```python
from build123d import *

# Parameters (mm, degrees)
CUT_EXTRUDE1_DEPTH = 1.5
CHAMFER1_SIZE      = 0.5


with BuildPart() as part:
    # Sketch2 → Revolve1 (revolve)
    with BuildSketch(Plane(origin=(0, 0, 0), x_dir=(1, 0, 0), z_dir=(0, 1, 0))):
        Polygon((-18, -4.5), (-11, -4.5), (-11, 0), (-5, 0), (-5, -5.4), (-11, -5.4), (-11, -15.4), (-18, -15.4), align=None)
    revolve(axis=Axis((0, 0, 0), (0, 0, 1)))

    # Sketch3 → Cut-Extrude1 (cut)
    with BuildSketch(Plane(origin=(0, 0, 0), x_dir=(-1, 0, 0), z_dir=(0, 0, -1))):
        with BuildLine():
            Line((1.25, 10.940968966), (1.25, 4.841229183))
            ThreePointArc((1.25, 4.841229183), (0, 5), (-1.25, 4.841229183))
            Line((-1.25, 4.841229183), (-1.25, 10.940968966))
            ThreePointArc((-1.25, 10.940968966), (0, 11.012143385), (1.25, 10.940968966))
        make_face()
        with BuildLine():
            Line((1.25, -4.841229183), (1.25, -10.940968966))
            ThreePointArc((1.25, -10.940968966), (0, -11.012143385), (-1.25, -10.940968966))
            Line((-1.25, -10.940968966), (-1.25, -4.841229183))
            ThreePointArc((-1.25, -4.841229183), (0, -5), (1.25, -4.841229183))
        make_face()
    extrude(amount=-CUT_EXTRUDE1_DEPTH, mode=Mode.SUBTRACT)

    # Chamfer1
    chamfer1_edges = [part.edges().sort_by_distance(p)[0] for p in [
        (11, 0, 0),
        (-8.20822758, -7.322909258, 0),
        (18, 0, 15.4),
        (18, 0, 4.5),
        (5, 0, 5.4),
        (11, 0, 15.4),
    ]]
    chamfer(chamfer1_edges, length=CHAMFER1_SIZE)


solid = part.part
```
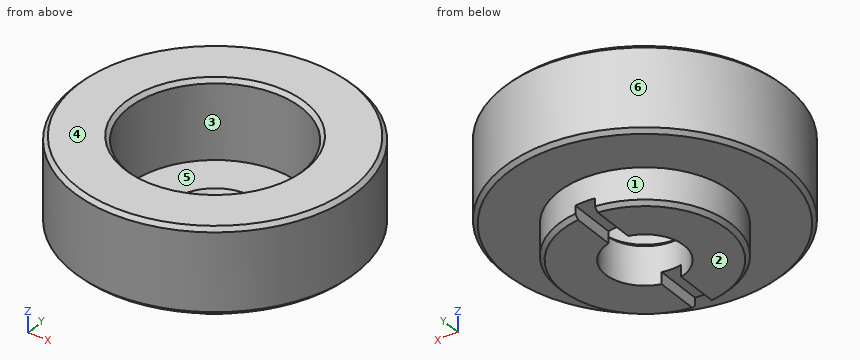
Read the model definition and answer for the solid it produces. Units are mm, in the model's axes. Face numbers are marked on the shaded views. A direction names the side the tool comes from. Give positions to 0.01 mm unless a question says otherwise; leave off trailing zeros. Order: outer loops, then holes, each group sorted by start corner. A loop starts at its lowest first (then second) coordinate and runs counter-clockwise, first axis right, second up.
(1) Find section A-A (y = 0). Give the vertices of the cut face in (x, z), plus the area to 3 significant figures.
(2) For a pull along X with two mould halves and no side action, classify the marked faces 4, 5 and 6 as released by +X, released by -X, zero draft, split by the parting line, or undercut.
(3) Find section B-B (x = 0). Give the vertices of the cut face in (y, z), plus the area to 3 significant figures.
(4) For the marked faces 1, 2 and 3, determine the directions among +Z, -Z, +X, -X, +Y, -Y from which every point of the face is accessible in a straight line to the end or side of a thin tool.
(5) Find section C-C (z = 13.5). Give the vertices of the cut face in (x, y), plus the area to 3 significant figures.
(6) Given pin 1 (0.5 mm diameter, centred on y = 8.5, z = 0.5, fed in from -X); pin 2 (0.8 mm diameter, centred on x = 0, y = 7, fed in from -Z); pin 3 (0.5 mm diameter, centred on y = -8, z = 1, fed in from +X), each flat-ended and moving along its own axis, determine where each tip first touches the part or whether it passes through.
(7) Straight lines are drawn through the part: L1, parallel to X at y = 0, z = 11.5; L2, parallel to Y at x = 0, z = 3.95. For each, find the intervals that lie inside material, in ascending order.
Result sheet:
1. outline: (-18, 5) - (-17.5, 4.5) - (-11, 4.5) - (-11, 0.5) - (-10.5, 0) - (-5, 0) - (-5, 4.9) - (-5.5, 5.4) - (-11, 5.4) - (-11, 14.9) - (-11.5, 15.4) - (-17.5, 15.4) - (-18, 14.9) - close; (5, 0) - (10.5, 0) - (11, 0.5) - (11, 4.5) - (17.5, 4.5) - (18, 5) - (18, 14.9) - (17.5, 15.4) - (11.5, 15.4) - (11, 14.9) - (11, 5.4) - (5.5, 5.4) - (5, 4.9) - close
1. area: 216 mm2
2. face 4: zero draft
2. face 5: undercut
2. face 6: split by the parting line
3. outline: (-18, 5) - (-17.5, 4.5) - (-11, 4.5) - (-11, 1.5) - (-5, 1.5) - (-5, 4.9) - (-5.5, 5.4) - (-11, 5.4) - (-11, 14.9) - (-11.5, 15.4) - (-17.5, 15.4) - (-18, 14.9) - close; (5, 1.5) - (11, 1.5) - (11, 4.5) - (17.5, 4.5) - (18, 5) - (18, 14.9) - (17.5, 15.4) - (11.5, 15.4) - (11, 14.9) - (11, 5.4) - (5.5, 5.4) - (5, 4.9) - close
3. area: 198 mm2
4. face 1: -Z
4. face 2: -Z, +X, -X, +Y, -Y
4. face 3: +Z
5. outline: circle Ø36 at (0, 0); hole circle Ø22 at (0, 0)
5. area: 638 mm2
6. pin 1: stops at x = -7.28
6. pin 2: stops at z = 1.5
6. pin 3: stops at x = 7.81
7. L1: x = -18 to -11, 11 to 18
7. L2: y = -11 to -5, 5 to 11
